The drawing under review shows one solid part. Ordinate dimensions are in mm from its lowest x, y, z. A direction names the side the tool comes from. Give positions to 0.01 mm unless a question says otherwise; leave off trailing zeros. Write each loop counter-clockwise with the first axis right and the second up, starting at its lowest first coordinate (ties: lowest second). Pieces come first, ordered by that corner, then holes.
Q1. We need section C-C (y = 52.5). Write out the cut boundary in (x, z), then the cut area to 3 significant figures.
Q2. Insertion check: P1, Ø9, axis at x = 63.5, y = 53.5, coming from the +Z side; P2, Ø12, axis at x = 39.5, y = 85.5, coming from the +Z side; P3, Ø1, axis at x = 43, y = 38.5, coming from the -Z side; P4, Ø6.5, axis at y = 31.5, z = 28, coming from the +X side. Each pin has a flat end and moves straight along its axis. Give the tip position at first contact, or say it passes through.
Q3. Mouldability with a two-part tool opening along Z and no side actions: class the marked faces 3, 4 and 5 as released by +Z, released by -Z, zero draft, split by the parting line, or undercut.
Q4. We need section A-A (z = 60). Write out the cut boundary in (x, y), then the cut area to 3 significant figures.
Q5. For line 1 (X direction, y = 34, z = 60); line 2 (X direction, y = 13, z = 38); line 3 (Z direction, x = 71, y = 5.5), list the stretches that pass through material, from the lowest coordinate up.
Q6. We need section B-B (x = 60). Write out the cut boundary in (y, z), then the cut area to 3 significant figures.
Q7. We need section D-D (z = 108). Write out the cut boundary in (x, y), then the cut area to 3 significant figures.
Q8. Machinability: for the marked faces 1 and 2, which of the approach directions +Z, -Z, +X, -X, +Y, -Y give a long, thin tool a straight path to every point of the face, cutting with its end or side? Answer none if there is none.
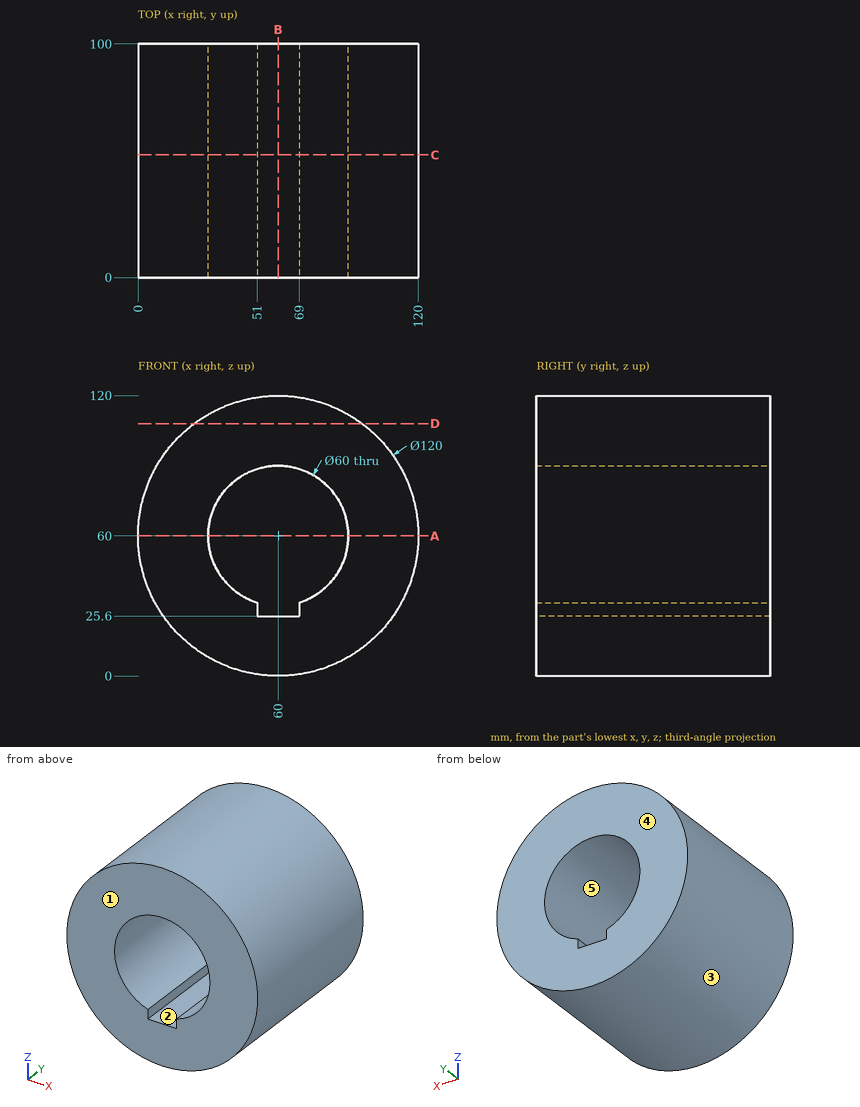
Computed:
1. outline: circle Ø120 at (60, 60); hole (51, 25.6) - (69, 25.6) - (69, 31.38) arc R30 ccw (long way) to (51, 31.38) - close
1. area: 8,390 mm2
2. P1: stops at z = 120
2. P2: stops at z = 118.22
2. P3: stops at z = 2.31
2. P4: stops at x = 112.66
3. face 3: split by the parting line
3. face 4: zero draft
3. face 5: undercut
4. outline: (0, 0) - (30, 0) - (30, 100) - (0, 100) - close; (90, 0) - (120, 0) - (120, 100) - (90, 100) - close
4. area: 6,000 mm2
5. line 1: x = 0 to 30, 90 to 120
5. line 2: x = 4.18 to 39.6, 80.4 to 115.82
5. line 3: z = 1.02 to 32.09, 87.91 to 118.98
6. outline: (0, 0) - (100, 0) - (100, 25.6) - (0, 25.6) - close; (0, 90) - (100, 90) - (100, 120) - (0, 120) - close
6. area: 5,560 mm2
7. outline: (24, 0) - (96, 0) - (96, 100) - (24, 100) - close
7. area: 7,200 mm2
8. face 1: +Z, -Z, +X, -X, -Y
8. face 2: +Y, -Y
